Solid Edge part; units mm, degrees
sketch "Sketch1" plane through (0, 0, 0) normal (0, 0, 1) x (1, 0, 0)
  circle A0 centre (0, 0) radius 9.525
extrude "Protrusion1" add sketch "Sketch1" along normal blind 7.9248
sketch "Sketch2" plane through (0, 0, 0) normal (0, 0, -1) x (0, 1, 0)
  circle A0 centre (0, 0) radius 6.35
extrude "Protrusion2" add sketch "Sketch2" along normal blind 15.875
sketch "Sketch3" plane through (0, 0, -15.875) normal (0, 0, -1) x (0, 1, 0)
  circle A0 centre (0, 0) radius 4.7625
extrude "Protrusion3" add sketch "Sketch3" along normal blind 15.875
sketch "Sketch4" plane through (0, 0, 7.9248) normal (0, 0, 1) x (0, 1, 0)
  line L0 (-3.175, 1.7461) -> (0, 3.8287)
  line L1 (-3.175, -2.051) -> (-3.175, 1.7461)
  line L2 (-3.175, -2.051) -> (0, -3.8287)
  line L3 (3.175, -2.051) -> (0, -3.8287)
  line L4 (3.175, -2.051) -> (3.175, 1.7461)
  line L5 (3.175, 1.7461) -> (0, 3.8287)
extrude "Cutout1" cut sketch "Sketch4" against normal blind 3.9624
chamfer "Chamfer1" distance 0.7874 angle 45 1 edges at (0, -4.7625, -31.75)
properties part number "192405"
Build history of the part. All positions in model axes, mm. A direction names the side the tool comes from. Round coordinates to 2 decimals unless told otherwise and drop trailing zeros. Write each loop counter-clockwise with the first axis right and the second up, starting at its lowest first coordinate (ties: lowest second). Pieces come first, ordered by that corner, then holes. Notation, with made-up numbers: M 19,77 L 75,77 A23 ccw 75,97 Z; hole C -1,49.25 d8. An arc over 180 degrees is marked long. Answer as a JSON object with one key per item and string values. Group by question number.
(1) Drill centre lines: L1, parallel to Z at x = 2.5, y = 0; L2, parallel to Z at x = -3.25, y = -8.5; L3, parallel to X at y = -2, z = 4.5. Where is each one in solid material? Low to high.
(2) Cut at D-D (z = -1.5). Give the cut face in (x, y), and give its area (3 significant figures).
(3) Flat gauge pins, fed straight in: pin 1 (10 mm diameter, centred on y = -6.5, z = -12, fed in from +X); pin 2 (3 mm diameter, centred on y = -2, z = -2, fed in from +X); pin 3 (1 mm diameter, centred on x = 3.5, y = -5.5, fed in from -Z) (3 decimals). Where does each tip first touch, or does it go through?
(4) Cut at C-C (z = -20.5). Give the cut face in (x, y) (1 decimal).
(5) Which spindle directions (+Z, -Z, +X, -X, +Y, -Y) get a long thin tool onto all of the face, cutting with end or side? Do faces 4 (the flat face through (4, 0, 7.925)), 5 (the flat face through (2.927, -1.61, 5.971)), 6 (the flat face through (6.2, -2, 0)). Say none if no direction does.
(6) Mould opens along Y. For faces 1 (the cylindrical face through (6.2, -1.38, -7.83)), 2 (the flat face through (0, 3.175, 6)), 3 (the flat face through (-1, 5, -15.875)) say: pulls with the +Y half, pulls with the -Y half, needs draft (parallel to the pull), parting line crosses it, or undercut.
(7) Cut at A-A (z = 4.5). Give the cut face in (x, y) (3 decimals), and give its area (3 significant figures).
Responses:
{
 "1": {"L1": "z = -31.75 to 3.96", "L2": "z = 0 to 7.92", "L3": "x = -9.31 to -2.52, 2.71 to 9.31"},
 "2": {"outline": "C 0,0 d12.7", "area": "127 mm2"},
 "3": {"pin 1": "stops at x = 6.17", "pin 2": "stops at x = 6.33", "pin 3": "stops at z = -15.875"},
 "4": {"outline": "C 0,0 d9.5"},
 "5": {"face 4": "+Z, +X, -X, +Y, -Y", "face 5": "+Z", "face 6": "-Z"},
 "6": {"face 1": "parting line crosses it", "face 2": "undercut", "face 3": "needs draft"},
 "7": {"outline": "C 0,0 d19.05; hole M -3.829,0 L -1.746,-3.175 L 2.051,-3.175 L 3.829,0 L 2.051,3.175 L -1.746,3.175 Z", "area": "249 mm2"}
}
